from build123d import *

# Parameters (mm, degrees)
F0_R     = 4.5
F0_R_2   = 3.3
F1_DEPTH = 6.4
F2_DEPTH = 8.4
F4_COUNT = 23
F5_DEPTH = 2
F6_DEPTH = 5.85
F7_DEPTH = 7.07


with BuildPart() as f1:
    # F0 (on Top) → F1 (new body)
    with BuildSketch(Plane.XY):
        with BuildLine():
            ThreePointArc((0, 7.1100645757), (-4.3416356365, -3.3715710607), (6.14, 0.9700645757))
            ThreePointArc((6.14, 0.9700645757), (4.6187674474, 5.0156284755), (0.8088640824, 7.0565527994))
            ThreePointArc((0.8088640824, 7.0565527994), (0.4053161155, 7.0966720257), (0, 7.1100645757))
        make_face()
        with Locations((0, 0.9700645757)):
            Circle(F0_R, mode=Mode.SUBTRACT)
        with Locations((0, 0.9700645757)):
            Circle(F0_R)
        with Locations((0, 0.9700645757)):
            Circle(F0_R_2, mode=Mode.SUBTRACT)
        with BuildLine():
            ThreePointArc((0, 7.6100645757), (0.4051871433, 7.5976903481), (0.8088640824, 7.5606137863))
            Line((0.8088640824, 7.5606137863), (0.8088640824, 8.3760242635))
            ThreePointArc((0.8088640824, 8.3760242635), (0.4050310645, 8.4090463499), (0, 8.4200645757))
            Line((0, 8.4200645757), (0, 7.6100645757))
        make_face()
        with BuildLine():
            ThreePointArc((0, 7.1100645757), (0.4053161155, 7.0966720257), (0.8088640824, 7.0565527994))
            Line((0.8088640824, 7.0565527994), (0.8088640824, 7.5606137863))
            ThreePointArc((0.8088640824, 7.5606137863), (0.4051871433, 7.5976903481), (0, 7.6100645757))
            Line((0, 7.6100645757), (0, 7.1100645757))
        make_face()
        with BuildLine():
            ThreePointArc((0, 8.4200645757), (0.4050310645, 8.4090463499), (0.8088640824, 8.3760242635))
            Line((0.8088640824, 8.3760242635), (0.8088640824, 8.5771822228))
            ThreePointArc((0.8088640824, 8.5771822228), (0.405, 8.6093364651), (0, 8.6200645757))
            Line((0, 8.6200645757), (0, 8.4200645757))
        make_face()
    extrude(amount=F1_DEPTH)



with BuildPart() as f2:
    # F0 (on Top) → F2 (new body)
    with BuildSketch(Plane.XY):
        with BuildLine():
            ThreePointArc((0.8088640824, 7.0565527994), (4.6187674474, 5.0156284755), (6.14, 0.9700645757))
            ThreePointArc((6.14, 0.9700645757), (-4.3416356365, -3.3715710607), (0, 7.1100645757))
            Line((0, 7.1100645757), (0, 7.6100645757))
            ThreePointArc((0, 7.6100645757), (-4.6951890271, -3.7251244513), (6.64, 0.9700645757))
            ThreePointArc((6.64, 0.9700645757), (4.9729497035, 5.3699931259), (0.8088640824, 7.5606137863))
            Line((0.8088640824, 7.5606137863), (0.8088640824, 7.0565527994))
        make_face()
        with BuildLine():
            ThreePointArc((0, 7.1100645757), (0.4053161155, 7.0966720257), (0.8088640824, 7.0565527994))
            Line((0.8088640824, 7.0565527994), (0.8088640824, 7.5606137863))
            ThreePointArc((0.8088640824, 7.5606137863), (0.4051871433, 7.5976903481), (0, 7.6100645757))
            Line((0, 7.6100645757), (0, 7.1100645757))
        make_face()
    extrude(amount=F2_DEPTH)


with BuildPart() as f1_1:
    add(f1.part)

    add(f2.part)  # F4 merges F2
    # F4: F1 ×23 about axis
    f4_axis = Axis((0, 0.9700645757, -1.082088449), (0, 0, -1))
    for i in range(1, F4_COUNT):
        add(f1.part.rotate(f4_axis, i * 360 / F4_COUNT))

    # F0 (on Top) → F5 (join)
    with BuildSketch(Plane.XY):
        with BuildLine():
            ThreePointArc((0, 7.1100645757), (-4.3416356365, -3.3715710607), (6.14, 0.9700645757))
            ThreePointArc((6.14, 0.9700645757), (4.6187674474, 5.0156284755), (0.8088640824, 7.0565527994))
            ThreePointArc((0.8088640824, 7.0565527994), (0.4053161155, 7.0966720257), (0, 7.1100645757))
        make_face()
        with Locations((0, 0.9700645757)):
            Circle(F0_R, mode=Mode.SUBTRACT)
    extrude(amount=-F5_DEPTH)

    # F0 (on Top) → F6 (join)
    with BuildSketch(Plane.XY):
        with BuildLine():
            ThreePointArc((0.8088640824, 7.0565527994), (4.6187674474, 5.0156284755), (6.14, 0.9700645757))
            ThreePointArc((6.14, 0.9700645757), (-4.3416356365, -3.3715710607), (0, 7.1100645757))
            Line((0, 7.1100645757), (0, 7.6100645757))
            ThreePointArc((0, 7.6100645757), (-4.6951890271, -3.7251244513), (6.64, 0.9700645757))
            ThreePointArc((6.64, 0.9700645757), (4.9729497035, 5.3699931259), (0.8088640824, 7.5606137863))
            Line((0.8088640824, 7.5606137863), (0.8088640824, 7.0565527994))
        make_face()
        with BuildLine():
            ThreePointArc((0, 7.1100645757), (0.4053161155, 7.0966720257), (0.8088640824, 7.0565527994))
            Line((0.8088640824, 7.0565527994), (0.8088640824, 7.5606137863))
            ThreePointArc((0.8088640824, 7.5606137863), (0.4051871433, 7.5976903481), (0, 7.6100645757))
            Line((0, 7.6100645757), (0, 7.1100645757))
        make_face()
    extrude(amount=-F6_DEPTH)

    # F0 (on Top) → F7 (join)
    with BuildSketch(Plane.XY):
        with BuildLine():
            Line((0.8088640824, 8.3760242635), (0.8088640824, 7.5606137863))
            ThreePointArc((0.8088640824, 7.5606137863), (4.9729497035, 5.3699931259), (6.64, 0.9700645757))
            ThreePointArc((6.64, 0.9700645757), (-4.6951890271, -3.7251244513), (0, 7.6100645757))
            Line((0, 7.6100645757), (0, 8.4200645757))
            ThreePointArc((0, 8.4200645757), (-5.2679455198, -4.2978809441), (7.45, 0.9700645757))
            ThreePointArc((7.45, 0.9700645757), (5.54655467, 5.9438188211), (0.8088640824, 8.3760242635))
        make_face()
        with BuildLine():
            Line((0.8088640824, 8.5771822228), (0.8088640824, 8.3760242635))
            ThreePointArc((0.8088640824, 8.3760242635), (5.54655467, 5.9438188211), (7.45, 0.9700645757))
            ThreePointArc((7.45, 0.9700645757), (-5.2679455198, -4.2978809441), (0, 8.4200645757))
            Line((0, 8.4200645757), (0, 8.6200645757))
            ThreePointArc((0, 8.6200645757), (-5.4093668761, -4.4393023003), (7.65, 0.9700645757))
            ThreePointArc((7.65, 0.9700645757), (5.6881592027, 6.0854672857), (0.8088640824, 8.5771822228))
        make_face()
        with BuildLine():
            ThreePointArc((0, 7.6100645757), (0.4051871433, 7.5976903481), (0.8088640824, 7.5606137863))
            Line((0.8088640824, 7.5606137863), (0.8088640824, 8.3760242635))
            ThreePointArc((0.8088640824, 8.3760242635), (0.4050310645, 8.4090463499), (0, 8.4200645757))
            Line((0, 8.4200645757), (0, 7.6100645757))
        make_face()
        with BuildLine():
            ThreePointArc((0, 8.4200645757), (0.4050310645, 8.4090463499), (0.8088640824, 8.3760242635))
            Line((0.8088640824, 8.3760242635), (0.8088640824, 8.5771822228))
            ThreePointArc((0.8088640824, 8.5771822228), (0.405, 8.6093364651), (0, 8.6200645757))
            Line((0, 8.6200645757), (0, 8.4200645757))
        make_face()
    extrude(amount=-F7_DEPTH)


solid = f1_1.part
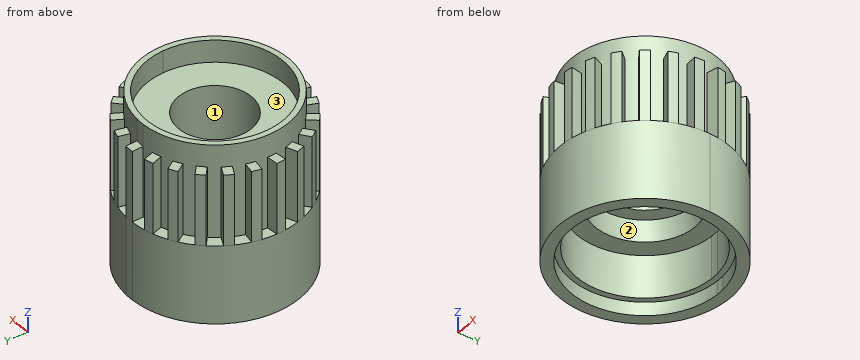
Check sheet for the modelled part. Datum: model origin and axes. Units: mm. Face numbers are marked on the shaded views. A direction names the side the tool comes from. Coordinates: 2 decimals unless noted, no trailing zeros.
Item 1: Scan lines: probe 1 along Y at (x, z) = (6, 2); probe 2 along Z at (x, y) = (-4, -4.5); probe 3 along Z at (x, y) = (2, 6). Record each from-to range of solid material in increasing order.
Numbers:
probe 1: y = -3.78 to -3.27, -2.02 to 4.08, 5.47 to 5.72
probe 2: z = -7.07 to 0
probe 3: z = -2 to 6.4
Item 2: Access from +Z, -Z, +X, -X, +Y, -Y to the whole of each face (thin tool, end or side, straight path). Record for the marked faces 1, 2 and 3.
Numbers:
face 1: +Z, -Z
face 2: -Z
face 3: +Z
Item 3: Depth check by flat-ended pin: pin 1 Ø3.5 at (x, y) = (-2.5, 3) entering from +Z; pin 2 Ø1 at (x, z) = (-3.5, -2) entering from -Y; pin 3 Ø1.5 at (x, z) = (1, 5) entering from -Y; pin 4 Ø4 at (x, y) = (2.5, 6) entering from -Z. Enter the tip coordinate at first touch or a pass-through.
Numbers:
pin 1: stops at z = 6.4
pin 2: stops at y = -6.07
pin 3: stops at y = -6.68
pin 4: stops at z = -7.07
